Read the model definition and answer for the solid it produces. Units are mm, in the model's axes. A direction names the side the tool comes from. Round coordinates to 2 decimals unless told otherwise and drop trailing zeros. Write each loop counter-clockwise with the first axis right and the second up, starting at its lowest first coordinate (ties: lowest second). Pieces come first, ordered by that corner, then holes. Notation, with made-up numbers: (25.25, 5) - (37.25, 5) arc R26 cw to (37.25, 20) - close; hole circle Ø5 at (30, 48). An arc over 180 degrees is marked (long way). One line per item, written item: value. Start each with the question number.
(1) A cutting plane is placed at C-C, the plane y = 3.25. Determine the outline of the cut face in (x, z).
(2) A cutting plane is placed at D-D, the plane z = -31.5. Determine the outline of the cut face in (x, y).
(3) For faces 1 (the face through (1.32, 10.99, -29.97)), 2 (the face through (9, 10, 29)), 3 (the face through (9.76, 15.94, 31)), determine the directions among +Z, -Z, +X, -X, +Y, -Y from which every point of the face is accessible in a straight line to the end or side of a thin tool.
(4) A cutting plane is placed at B-B, the plane z = 0. Determine the outline of the cut face in (x, y).
(5) Flat-ended cylindrical pins translate along their axes: pin 1 Ø2 at (y, z) = (8, -4) entering from -X; pin 2 Ø1.5 at (y, z) = (13, 34) entering from +X; pin 3 Ø12 at (y, z) = (17, -5) entering from +X; pin 4 Ø12 at (x, z) = (14.5, 11.5) entering from +Y. Find the tip coordinate at first contact, or state that the pin passes through.
(6) A cutting plane is placed at A-A, the plane x = 0. Determine the outline of the cut face in (y, z).
(7) The mould has two halves that part along X. Classify faces 4 (the face through (-31.3, 20, -9.6)), 5 (the face through (9.76, 4.93, 31)), 6 (the face through (-25.861, 9.86, -33.727)): +X half, -X half, draft (parallel to the pull), parting line (faces both ways), or undercut.
(8) Find the intervals of material crossed by L1, parallel to Z at x = -25.5, y = 2.5; L2, parallel to Z at x = 11.5, y = 13.5; L3, parallel to X at y = 11.65, z = 0, in increasing order.
from build123d import *

# Parameters (mm, degrees)
SKETCH1_R           = 42.5
SKETCH1_R_2         = 32.5
BOSS_EXTRUDE1_DEPTH = 20
SKETCH2_R           = 33
SKETCH2_R_2         = 30
BOSS_EXTRUDE2_DEPTH = 2


with BuildPart() as part:
    # Sketch1 → Boss-Extrude1 (new body)
    with BuildSketch(Plane(origin=(0, 0, 0), x_dir=(1, 0, 0), z_dir=(0, 1, 0))):
        with Locations(Location((0, 0, 0), (0, 0, 270))):
            Circle(SKETCH1_R)
        with Locations(Location((0, 0, 0), (0, 0, 270))):
            Circle(SKETCH1_R_2, mode=Mode.SUBTRACT)
    extrude(amount=BOSS_EXTRUDE1_DEPTH)

    # Sketch2 → Boss-Extrude2 (add)
    with BuildSketch(Plane(origin=(0, 10, 0), x_dir=(1, 0, 0), z_dir=(0, 1, 0))):
        Circle(SKETCH2_R)
        with Locations(Location((0, 0, 0), (0, 0, 270))):
            Circle(SKETCH2_R_2, mode=Mode.SUBTRACT)
    extrude(amount=BOSS_EXTRUDE2_DEPTH)


solid = part.part
Here are the results:
1. outline: circle Ø85 at (0, 0); hole circle Ø65 at (0, 0)
2. outline: (-28.53, 0) - (-8, 0) - (-8, 10) - (8, 10) - (8, 0) - (28.53, 0) - (28.53, 20) - (8, 20) - (8, 12) - (-8, 12) - (-8, 20) - (-28.53, 20) - close
3. face 1: +Y, -Y
3. face 2: -Y
3. face 3: +Y
4. outline: (-42.5, 0) - (-32.5, 0) - (-32.5, 10) - (-30, 10) - (-30, 12) - (-32.5, 12) - (-32.5, 20) - (-42.5, 20) - close; (30, 10) - (32.5, 10) - (32.5, 0) - (42.5, 0) - (42.5, 20) - (32.5, 20) - (32.5, 12) - (30, 12) - close
5. pin 1: x = -42.39
5. pin 2: x = 26.47
5. pin 3: x = 42.5
5. pin 4: through
6. outline: (0, -42.5) - (20, -42.5) - (20, -32.5) - (12, -32.5) - (12, -30) - (10, -30) - (10, -32.5) - (0, -32.5) - close; (0, 32.5) - (10, 32.5) - (10, 30) - (12, 30) - (12, 32.5) - (20, 32.5) - (20, 42.5) - (0, 42.5) - close
7. face 4: draft
7. face 5: undercut
7. face 6: parting line
8. L1: -34 to -20.15, 20.15 to 34
8. L2: -40.91 to -30.4, 30.4 to 40.91
8. L3: -42.5 to -30, 30 to 42.5
